Here's the drawing with two shaded views (mm, measured from the low corner). I have some questions. A direction names the side the tool comes from. Round coordinates to 2 decimals unless told otherwise and drop trailing zeros. Write each loop counter-clockwise with the first axis right and the second up, starting at its lowest first coordinate (ties: lowest second). Pieces come first, ordered by that corner, then holes. Notation, with made-up numbers: M 3.5,76 L 62.5,76 A32 cw 62.5,103 Z; hole C 65.25,-9.75 d2. An arc over 180 degrees is marked long. Answer as a JSON object with one key per item and string values. Group by question number.
1) Please list where this line runs through material, in increasing order: L1, parallel to X at y = 22.5, z = 99. Write a range as [from, to].
2) If we mould it in two halves opening along Y, with no side actions, what happens to the marked faces 1, 2 and 3? For each: +Y half, -Y half, draft (parallel to the pull), parting line (faces both ways), or undercut.
3) Suppose I cut it at B-B, the plane z = 86. Write out the boundary of the cut face in (x, y), and give its area (3 significant figures).
4) Suppose I cut it at A-A, the plane x = 16.5. Write out the boundary of the cut face in (y, z).
5) On a 3-axis mill with a long thin cutter (end or side, diameter ignored), from which of +Z, -Z, +X, -X, +Y, -Y can I reach the whole of each face in a straight line? I mean the marked faces 4 and 5. Say none if no direction works.
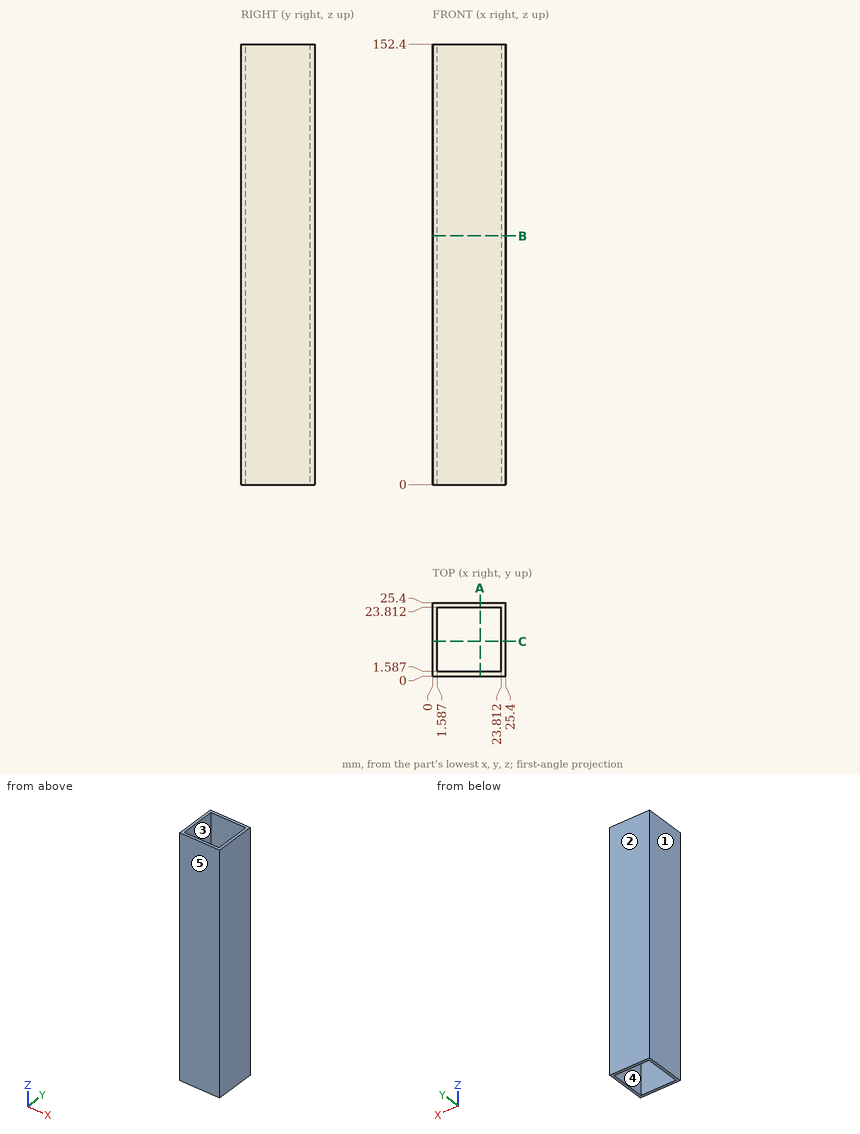
Results:
{
 "1": {"L1": "[0, 1.59], [23.81, 25.4]"},
 "2": {"face 1": "draft", "face 2": "+Y half", "face 3": "undercut"},
 "3": {"outline": "M 0,0 L 25.4,0 L 25.4,25.4 L 0,25.4 Z; hole M 1.59,1.59 L 23.81,1.59 L 23.81,23.81 L 1.59,23.81 Z", "area": "151 mm^2"},
 "4": {"outline": "M 0,0 L 1.59,0 L 1.59,152.4 L 0,152.4 Z; M 23.81,0 L 25.4,0 L 25.4,152.4 L 23.81,152.4 Z"},
 "5": {"face 4": "+Z, -Z", "face 5": "+Z, -Z, +X, -X, -Y"}
}
